Part model, mm, in its own coordinate system. Face numbers are marked on the shaded views. A direction names the side the tool comes from. Give positions to 0.01 mm unless a question says otherwise; leave off trailing zeros. Write each loop counter-clockwise with the first axis right and the second up, starting at its lowest first coordinate (ties: lowest second). Pieces come first, ordered by that corner, then holes.
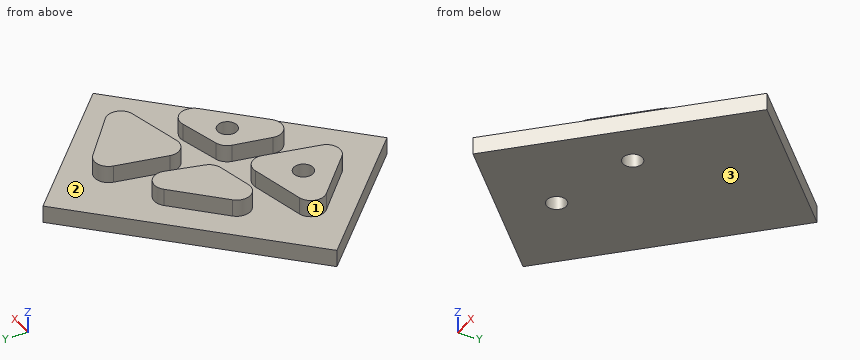
```python
from build123d import *

# Parameters (mm, degrees)
BOSS_EXTRUDE1_DEPTH     = 6.35
BOSS_EXTRUDE2_DEPTH     = 6.35
FILLET1_R               = 5.08
SKETCH3_R               = 3.556
CUT_EXTRUDE1_DEPTH      = 1.0000001
CUT_EXTRUDE1_DEPTH_BACK = 13.7


with BuildPart() as part:
    # Sketch1 → Boss-Extrude1 (new body)
    with BuildSketch(Plane.XY):
        Polygon((187.286286244, -255.536232765), (255.536232765, -187.286286244), (300.43751337, -232.18756685), (232.18756685, -300.43751337), align=None)
    extrude(amount=BOSS_EXTRUDE1_DEPTH)

    # Sketch2 → Boss-Extrude2 (add)
    with BuildSketch(Plane(origin=(-122.999277868, -379.350906339, 6.35), x_dir=(1, 0, 0), z_dir=(0, 0, 1))):
        Polygon((358.652446232, 129.843073159), (361.187345435, 130.431571088), (353.631906688, 99.023102123), (352.465526746, 94.616733593), (347.736029271, 99.326506792), (324.454742757, 121.903791925), align=None)
        Polygon((369.84495619, 105.077454433), (362.389303407, 97.597844709), (364.454204898, 107.026485871), (369.687373927, 130.92189838), (389.915729798, 136.377665107), (404.528274707, 139.872219424), align=None)
        Polygon((380.244489791, 174.237534533), (380.323081857, 174.55732413), (406.948495143, 150.901624736), (409.197553318, 148.774137273), (405.612483177, 147.90877996), (372.317989901, 139.872219424), align=None)
        Polygon((371.079053541, 165.746977866), (363.278943376, 137.878777762), (341.260989988, 132.802884769), (330.489965122, 130.230836291), (365.380288676, 164.810357377), (373.055677454, 172.41737391), align=None)
    extrude(amount=BOSS_EXTRUDE2_DEPTH)

    # Fillet1
    fillet1_edges = [part.edges().sort_by_distance(p)[0] for p in [
        (250.056399586, -206.933532429, 9.525),
        (257.323803989, -204.79358221, 9.525),
        (286.19827545, -230.576769066, 9.525),
        (249.318712034, -239.478686915, 9.525),
        (239.390025539, -281.753061631, 9.525),
        (246.688096059, -248.429007959, 9.525),
        (281.528996839, -239.478686915, 9.525),
        (201.455464889, -257.447114414, 9.525),
        (238.188067567, -248.919335251, 9.525),
        (207.490687255, -249.120070049, 9.525),
        (240.279665508, -241.472128577, 9.525),
        (229.466248878, -284.734172747, 9.525),
    ]]
    fillet(fillet1_edges, radius=FILLET1_R)

    # Sketch3 → Cut-Extrude1 (cut, two sides)
    with BuildSketch(Plane.XY.offset(12.7)) as cut_extrude1_sk:
        with Locations((254.802658362, -254.853889617)):
            Circle(SKETCH3_R)
        with Locations((222.616120289, -263.9547)):
            Circle(SKETCH3_R)
    extrude(amount=CUT_EXTRUDE1_DEPTH, mode=Mode.SUBTRACT)
    extrude(cut_extrude1_sk.sketch, amount=-CUT_EXTRUDE1_DEPTH_BACK, mode=Mode.SUBTRACT)


solid = part.part
```
1) Saw through at A-A, the plane z = 8.75. Count the separate pieces of the cut face and the enclosed holes in it, then the cut area to 3 significant figures.
Answers follow:
separate pieces: 4
enclosed holes: 2
area: 1,880 mm2
2) Wall check: L1, parallel to X at y = -261, z = 9.5; L2, parallel to Y at x = 222, z = 11.5; L3, parallel to Z at x = 271.5, y = -247. Give the ranges that are in metal, low to high.
Answers follow:
L1: x = 206.65 to 220.64, 224.59 to 235.28, 243.94 to 260.08
L2: y = -277.37 to -267.46, -260.45 to -252.68, -244.77 to -234.74
L3: z = 0 to 6.35
3) Pin check, flat tips, straight feed: pin 1 Ø6 at (x, z) = (219.5, 6.5) entering from +Y; pin 2 Ø1.5 at (y, z) = (-235.5, 4) entering from +X; pin 3 Ø3 at (x, z) = (228, 3) entering from +Y. Stop position of each tip, or through.
Answers follow:
pin 1: stops at y = -220.33
pin 2: stops at x = 297.88
pin 3: stops at y = -213.32
4) 3-axis set-ups, long thin cutter, end or side, ignore diameter. For the marked faces 1, 2 and 3: which of +Z, -Z, +X, -X, +Y, -Y reach the whole face in a straight line?
Answers follow:
face 1: +Z, -X
face 2: +Z
face 3: -Z, +X, -X, +Y, -Y
5) Saw through at C-C, the plane z = 1.5. Write the cut outline in (x, y), then the cut area to 3 significant figures.
Answers follow:
outline: (187.29, -255.54) - (232.19, -300.44) - (300.44, -232.19) - (255.54, -187.29) - close; hole circle Ø7.11 at (222.62, -263.95); hole circle Ø7.11 at (254.8, -254.85)
area: 6,050 mm2
6) Saw through at D-D, the plane x = 283.5. Write the cut outline in (y, z), then the cut area to 3 significant figures.
Answers follow:
outline: (-249.13, 0) - (-215.25, 0) - (-215.25, 6.35) - (-249.13, 6.35) - close
area: 215 mm2
7) Saw through at B-B, the plane y = -214.5. Write the cut outline in (x, z), then the cut area to 3 significant figures.
Answers follow:
outline: (228.32, 0) - (282.75, 0) - (282.75, 6.35) - (268.25, 6.35) - (268.25, 12.7) - (255.08, 12.7) - (255.08, 6.35) - (228.32, 6.35) - close
area: 429 mm2
